Read the model definition and answer for the solid it produces. Units are mm, in the model's axes. A direction names the side the tool comes from. Coordinates: 2 decimals unless noted, no trailing zeros. Write each loop counter-clockwise with the first axis right and the second up, starting at its lowest first coordinate (ties: lowest second). Pieces come first, ordered by that corner, then holes. Notation, with made-up numbers: (-18, 27.5) -> (39, 27.5) arc R17 cw to (39, 51.5) -> close; hole circle Ø1 at (-25.5, 88). An arc over 180 degrees is marked (long way). Use CSV: the item, a comma, the result in double quotes.
from build123d import *

# Parameters (mm, degrees)
BOSS_EXTRUDE1_DEPTH = 390.3
BOSS_EXTRUDE2_DEPTH = 4.3
SKETCH3_W           = 8.6
SKETCH3_H           = 70
CUT_EXTRUDE1_DEPTH  = 10


with BuildPart() as part:
    # Sketch1 → Boss-Extrude1 (new body)
    with BuildSketch(Plane.XY):
        Polygon((-30, 0), (-25.7, 0), (-25.7, 20.7), (25.7, 20.7), (25.7, 0), (30, 0), (30, 25), (-30, 25), align=None)
    extrude(amount=BOSS_EXTRUDE1_DEPTH)

    # Sketch2 → Boss-Extrude2 (add)
    with BuildSketch(Plane(origin=(30, 0, 0), x_dir=(0, 0, -1), z_dir=(1, 0, 0))):
        Polygon((-306, -12.31), (0, 0), (-390.3, 0), (-390.3, -12.31), align=None)
    boss_extrude2 = extrude(amount=-BOSS_EXTRUDE2_DEPTH)

    # Mirror1: Boss-Extrude2 across plane
    add(boss_extrude2.mirror(Plane(origin=(0, 0, 0), x_dir=(0, 0, 1), z_dir=(1, 0, 0))))

    # Sketch3 → Cut-Extrude1 (cut)
    with BuildSketch(Plane(origin=(0, 25, 0), x_dir=(1, 0, 0), z_dir=(0, 1, 0))):
        with Locations((0, -35)):
            Rectangle(SKETCH3_W, SKETCH3_H)
    extrude(amount=-CUT_EXTRUDE1_DEPTH, mode=Mode.SUBTRACT)


solid = part.part
1. Find the intervals of material crossed by line 1 along X through (y, z) = (-9, 252.5); line 2 along Y through (x, z) = (-20, 261); line 3 along Y through (x, z) = (26, 240), in increasing order.
Solutions:
line 1,"x = -30 to -25.7, 25.7 to 30"
line 2,"y = 20.7 to 25"
line 3,"y = -9.65 to 25"
2. A cutting plane is placed at B-B (z = 322). Give the vertices of the cut face in (x, y).
Solutions:
outline,"(-30, -12.31) -> (-25.7, -12.31) -> (-25.7, 20.7) -> (25.7, 20.7) -> (25.7, -12.31) -> (30, -12.31) -> (30, 25) -> (-30, 25) -> close"
3. A cutting plane is placed at D-D (z = 282). Give the vertices of the cut face in (x, y), and give its area (3 significant figures).
Solutions:
outline,"(-30, -11.34) -> (-25.7, -11.34) -> (-25.7, 20.7) -> (25.7, 20.7) -> (25.7, -11.34) -> (30, -11.34) -> (30, 25) -> (-30, 25) -> close"
area,"534 mm^2"
4. A cutting plane is placed at C-C (x = 20). Give the vertices of the cut face in (y, z), and give its area (3 significant figures).
Solutions:
outline,"(20.7, 0) -> (25, 0) -> (25, 390.3) -> (20.7, 390.3) -> close"
area,"1,680 mm^2"
5. A cutting plane is placed at A-A (y = 5). Give the vertices of the cut face in (x, z).
Solutions:
outline,"(-30, 0) -> (-25.7, 0) -> (-25.7, 390.3) -> (-30, 390.3) -> close; (25.7, 0) -> (30, 0) -> (30, 390.3) -> (25.7, 390.3) -> close"
6. Each of these flat-tipped pins is pushed along its axis until it touches: pin 1 Ø12 at (x, z) = (24, 141.5) entering from -Y; pin 2 Ø5 at (x, z) = (-18.5, 277) entering from -Y; pin 3 Ø1.3 at (x, y) = (1, 24) entering from -Z; pin 4 Ø10 at (x, y) = (-17, 12) entering from -Z. Where does it stop, or does it pass through?
Solutions:
pin 1,"stops at y = -5.92"
pin 2,"stops at y = 20.7"
pin 3,"stops at z = 70"
pin 4,"passes through"
7. For a pull along X with two mould halves and no side action, classify faces 3 (the flat face through (0, 22, 390.3)), 4 (the flat face through (30, 7, 198)), 5 (the flat face through (25.7, 8, 198)), 6 (the flat face through (-30, 7, 198)) as pulls with the +X half, pulls with the -X half, needs draft (parallel to the pull), parting line crosses it, or undercut.
Solutions:
face 3,"needs draft"
face 4,"pulls with the +X half"
face 5,"undercut"
face 6,"pulls with the -X half"
8. A tool of negligible diameter and unlimited length cuts with its end or side. For faces 1 (the flat face through (-25.7, 8, 198)), 2 (the flat face through (21, 23, 0)), from which of +Z, -Z, +X, -X, +Y, -Y can it reach the whole face along a straight path? Write none if from no direction.
Solutions:
face 1,"+Z, -Z, -Y"
face 2,"-Z, +X, -X, +Y, -Y"
